```python
from build123d import *

# Parameters (mm, degrees)
SKETCH4_R           = 1.905
BOSS_EXTRUDE1_DEPTH = 101.6
SKETCH5_R           = 1.905
BOSS_EXTRUDE2_DEPTH = 75.692
SKETCH7_R           = 1.905
BOSS_EXTRUDE3_DEPTH = 88.9


with BuildPart() as part:
    # Sketch4 → Boss-Extrude1 (new body)
    with BuildSketch(Plane.XY):
        Circle(SKETCH4_R)
    extrude(amount=BOSS_EXTRUDE1_DEPTH)

    # Sketch5 → Boss-Extrude2 (add)
    with BuildSketch(Plane(origin=(0, 0, 0), x_dir=(0, 0, -1), z_dir=(1, 0, 0))):
        with Locations((-101.6, 0)):
            Circle(SKETCH5_R)
    extrude(amount=BOSS_EXTRUDE2_DEPTH)

    # Sketch6 → Revolve1 (revolve)
    with BuildSketch(Plane.ZY):
        with BuildLine():
            Line((101.6, 1.905), (101.6, -1.905))
            ThreePointArc((101.6, -1.905), (103.505, 0), (101.6, 1.905))
        make_face()
    revolve(axis=Axis((0, 1.905, 101.6), (0, -1, 0)))

    # Sketch7 → Boss-Extrude3 (add)
    with BuildSketch(Plane(origin=(0, 0, 0), x_dir=(1, 0, 0), z_dir=(0, 1, 0))):
        with Locations((75.692, -101.6)):
            Circle(SKETCH7_R)
    extrude(amount=-BOSS_EXTRUDE3_DEPTH)

    # Sketch8 → Revolve2 (revolve)
    with BuildSketch(Plane(origin=(0, 0, 0), x_dir=(1, 0, 0), z_dir=(0, 1, 0))):
        with BuildLine():
            Line((75.692, -99.695), (75.692, -103.505))
            ThreePointArc((75.692, -103.505), (77.597, -101.6), (75.692, -99.695))
        make_face()
    revolve(axis=Axis((75.692, 0, 99.695), (0, 0, 1)))


solid = part.part
```
Could you check a few things on this model? Use its own coordinates, in mm. A direction names the side the tool comes from. Coordinates: 2 decimals unless noted, no trailing zeros. Loops run counter-clockwise (first coordinate to the right, second up) from the corner with the lowest first, then second, coordinate; pieces in that order, holes last.
1) Imagine slicing it at B-B (x = 59.5). List the corners of the cut face in (y, z) for me (3 decimals), and give its area (3 significant figures).
Reported:
outline: circle Ø3.81 at (0, 101.6)
area: 11.4 mm2
2) Imagine slicing it at A-A (z = 88). List the corners of the cut face in (x, y) for me (3 decimals), and give its area (3 significant figures).
Reported:
outline: circle Ø3.81 at (0, 0)
area: 11.4 mm2
3) Thinking about a two-plate mould opening in Y: for faces 1 (the face through (76, -88.9, 102)), 2 (the face through (37.316, 0.084, 103.503)), 3 (the face through (77.45, -43.83, 102.33)), which applies, released by +Y, released by -Y, zero draft, split by the parting line, or undercut?
Reported:
face 1: released by -Y
face 2: split by the parting line
face 3: zero draft
4) Which directions (+Z, -Z, +X, -X, +Y, -Y) give clear straight access to the entire face, cutting with the end or side of a thin tool? Please do faces 4 (the face through (-0.41, -1.86, 50.09)), 5 (the face through (0, 0, 0)).
Reported:
face 4: -Z
face 5: -Z, +X, -X, +Y, -Y
